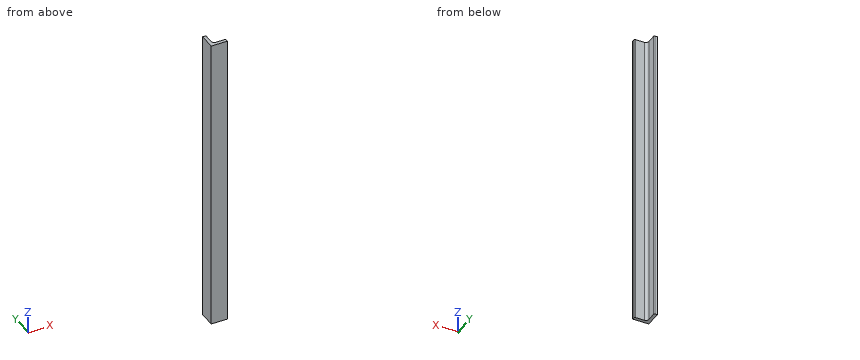
```python
from build123d import *

# Parameters (mm, degrees)
EXTRUDE_1_DEPTH = 372


with BuildPart() as part:
    # Эскиз1 → Бобышка-Вытянуть1 (new body)
    with BuildSketch(Plane.XY):
        with BuildLine():
            Line((-7.5, 12.5), (-7.5, -7.5))
            Line((-7.5, -7.5), (12.5, -7.5))
            Line((12.5, -7.5), (12.5, -4.7))
            ThreePointArc((12.5, -4.7), (12.148528137, -3.851471863), (11.3, -3.5))
            Line((11.3, -3.5), (0, -3.5))
            ThreePointArc((0, -3.5), (-2.474873734, -2.474873734), (-3.5, 0))
            Line((-3.5, 0), (-3.5, 11.3))
            ThreePointArc((-3.5, 11.3), (-3.851471863, 12.148528137), (-4.7, 12.5))
            Line((-4.7, 12.5), (-7.5, 12.5))
        make_face()
    extrude(amount=EXTRUDE_1_DEPTH)


solid = part.part
```
Verification items for the finished model (mm, model axes). Coordinates: 2 decimals unless noted, no trailing zeros. Order: outer loops, then holes, each group sorted by start corner. A loop starts at its lowest first (then second) coordinate and runs counter-clockwise, first axis right, second up. Notation, with made-up numbers: (58, 17) -> (72, 17) arc R21 ccw to (72, 54) -> close; hole circle Ø9 at (-8.5, -19.75). An arc over 180 degrees is marked (long way). Answer as CSV lines item,"result". Start each with the question number.
1) Cross-section at B-B, the plane y = 3.5. Record the boundary of the cut face in (x, z).
2) Cross-section at A-A, the plane z = 97.5. Record the boundary of the cut face in (x, y), then the cut area to 3 significant figures.
3) Gauge pin test, flat ends, axial feed: pin 1 Ø4 at (y, z) = (9, 83) entering from +X; pin 2 Ø3.5 at (x, z) = (6, 127.5) entering from +Y; pin 3 Ø12 at (x, z) = (3.5, 102) entering from +Y. Record the tip position at first contact, or that the pin passes through.
4) Material ranges on L1, parallel to Y at x = 6, z = 69.5; L2, parallel to X at y = -2.5, z = 335.5, recorded low to high. Write a range as [from, to].
Conclusion:
1,outline,"(-7.5, 0) -> (-3.5, 0) -> (-3.5, 372) -> (-7.5, 372) -> close"
2,outline,"(-7.5, -7.5) -> (12.5, -7.5) -> (12.5, -4.7) arc R1.2 ccw to (11.3, -3.5) -> (0, -3.5) arc R3.5 cw to (-3.5, 0) -> (-3.5, 11.3) arc R1.2 ccw to (-4.7, 12.5) -> (-7.5, 12.5) -> close"
2,area,"146 mm²"
3,pin 1,"stops at x = -3.5"
3,pin 2,"stops at y = -3.5"
3,pin 3,"stops at y = -2.45"
4,L1,"y = [-7.5, -3.5]"
4,L2,"x = [-7.5, -2.45]"
